Verification items for the finished model (mm, model axes). A direction names the side the tool comes from. Round coordinates to 2 decimals unless told otherwise and drop trailing zeros. Loops run counter-clockwise (first coordinate to the right, second up) from the corner with the lowest first, then second, coordinate; pieces in that order, holes last. Notation, with made-up numbers: M 84,-24 L 94,-24 A13 cw 94,-2 Z; hole C -12,64 d9. An arc over 180 degrees is marked long. One line per item, written item: value.
from build123d import *

# Parameters (mm, degrees)
SKETCH_1_W          = 23.4
SKETCH_1_H          = 12
SKETCH_1_R          = 1.75
SKETCH_1_R_2        = 1.6
SKETCH_1_R_3        = 1.15
EXTRUDE_1_DEPTH     = 1
EXTRUDE_START       = 1
SKETCH_1_4_W        = 23.4
SKETCH_1_4_H        = 12
EXTRUDE_2_DEPTH     = 3.1
SKETCH_3_R          = 0.35
CUT_EXTRUDE_3_DEPTH = 2
SKETCH_3_3_R        = 1
CUT_EXTRUDE_4_DEPTH = 1
SKETCH_3_4_R        = 0.8
CUT_EXTRUDE_5_DEPTH = 27.615221209


with BuildPart() as part:
    # 草图1 → 凸台-拉伸1 (new body)
    with BuildSketch(Plane(origin=(0, 0, 0), x_dir=(1, 0, 0), z_dir=(0, 1, 0))):
        with Locations((11.7, -6)):
            Rectangle(SKETCH_1_W, SKETCH_1_H)
        with Locations(Location((9.270831301, -3.4, 0), (0, 0, 270))):
            Circle(SKETCH_1_R, mode=Mode.SUBTRACT)
        with Locations(Location((9.270831301, -8.6, 0), (0, 0, 270))):
            Circle(SKETCH_1_R, mode=Mode.SUBTRACT)
        with Locations(Location((12.695740059, -6, 0), (0, 0, 270))):
            Circle(SKETCH_1_R_2, mode=Mode.SUBTRACT)
        with Locations(Location((18.395740059, -6, 0), (0, 0, 270))):
            Circle(SKETCH_1_R_3, mode=Mode.SUBTRACT)
    extrude(amount=EXTRUDE_1_DEPTH)

    # 草图1<4> → 凸台-拉伸2 (add)
    with BuildSketch(Plane(origin=(0, 0, 0), x_dir=(1, 0, 0), z_dir=(0, 1, 0)).offset(EXTRUDE_START)):
        with Locations((11.7, -6)):
            Rectangle(SKETCH_1_4_W, SKETCH_1_4_H)
        with BuildLine():
            ThreePointArc((9.300586178, -5.149747024), (7.876973085, -2.341860465), (10.964181547, -2.958338428))
            ThreePointArc((10.964181547, -2.958338428), (13.1957667, -2.53590223), (15.21679269, -3.572183362))
            ThreePointArc((15.21679269, -3.572183362), (19.67718661, -2.210818725), (22.395740059, -6))
            ThreePointArc((22.395740059, -6), (19.67718661, -9.789181275), (15.21679269, -8.427816638))
            ThreePointArc((15.21679269, -8.427816638), (13.1957667, -9.46409777), (10.964181547, -9.041661572))
            ThreePointArc((10.964181547, -9.041661572), (7.876973085, -9.658139535), (9.300586178, -6.850252976))
            ThreePointArc((9.300586178, -6.850252976), (9.195740059, -6), (9.300586178, -5.149747024))
        make_face(mode=Mode.SUBTRACT)
    extrude(amount=EXTRUDE_2_DEPTH)

    # 草图3 → 切除-拉伸3 (cut)
    with BuildSketch(Plane(origin=(0, 4.1, 0), x_dir=(1, 0, 0), z_dir=(0, 1, 0))):
        with Locations(Location((2.419185522, -2.108925173, 0), (0, 0, 270))):
            Circle(SKETCH_3_R)
        with Locations(Location((14.983521503, -1.209932246, 0), (0, 0, 270))):
            Circle(SKETCH_3_R)
        with Locations(Location((14.983521503, -10.376111281, 0), (0, 0, 270))):
            Circle(SKETCH_3_R)
        with Locations(Location((5.314681037, -6.384388153, 0), (0, 0, 270))):
            Circle(SKETCH_3_R)
    extrude(amount=-CUT_EXTRUDE_3_DEPTH, mode=Mode.SUBTRACT)

    # 草图3<3> → 切除-拉伸4 (cut)
    with BuildSketch(Plane(origin=(0, 4.1, 0), x_dir=(1, 0, 0), z_dir=(0, 1, 0))):
        with Locations(Location((1.568943185, -5.332489754, 0), (0, 0, 270))):
            Circle(SKETCH_3_3_R)
        with Locations(Location((2.419185522, -9.817518082, 0), (0, 0, 270))):
            Circle(SKETCH_3_3_R)
        with Locations((21.143175994, -2.108925173)):
            Circle(SKETCH_3_3_R)
        with Locations((21.143175994, -9.817518082)):
            Circle(SKETCH_3_3_R)
    extrude(amount=-CUT_EXTRUDE_4_DEPTH, mode=Mode.SUBTRACT)

    # 草图3<4> → 切除-拉伸5 (cut, through all)
    with BuildSketch(Plane(origin=(0, 4.1, 0), x_dir=(1, 0, 0), z_dir=(0, 1, 0))):
        with Locations(Location((1.568943185, -5.332489754, 0), (0, 0, 270))):
            Circle(SKETCH_3_4_R)
        with Locations(Location((21.143175994, -2.108925173, 0), (0, 0, 270))):
            Circle(SKETCH_3_4_R)
        with Locations(Location((2.419185522, -9.817518082, 0), (0, 0, 270))):
            Circle(SKETCH_3_4_R)
        with Locations(Location((21.143175994, -9.817518082, 0), (0, 0, 270))):
            Circle(SKETCH_3_4_R)
    extrude(amount=-CUT_EXTRUDE_5_DEPTH, mode=Mode.SUBTRACT)


solid = part.part
(1) Sectioned sample at A-A on z = 8. Enter the section's corners in (x, y).
Completed:
outline: M 0,0 L 7.63,0 L 7.63,4.1 L 0,4.1 Z; M 10.91,0 L 23.4,0 L 23.4,4.1 L 21.86,4.1 L 21.86,1 L 10.91,1 Z
(2) Mould release check, pull along X, two halves, no side actions. Record for faces 1 (the face through (2.96, 1.57, 9.23)), 2 (the face through (12, 2, 12)): +X half, -X half, draft (parallel to the pull), parting line (faces both ways), or undercut.
Completed:
face 1: undercut
face 2: draft
(3) Depth check by flat-ended pin: pin 1 Ø4 at (x, z) = (17.5, 7) entering from +Y. Enter the tip coordinate at first touch or a pass-through.
Completed:
pin 1: stops at y = 1
(4) Sectioned sample at B-B on x = 18. Enter the section's corners in (y, z), and give its area (3 significant figures).
Completed:
outline: M 0,0 L 4.1,0 L 4.1,2.02 L 1,2.02 L 1,4.92 L 0,4.92 Z; M 0,7.08 L 1,7.08 L 1,9.98 L 4.1,9.98 L 4.1,12 L 0,12 Z
area: 22.4 mm^2
(5) Thickness scan on L1, parallel to X at y = 0.45, z = 6; L2, parallel to Z at x = 8, y = 0.35; L3, parallel to Z at x = 7.75, y = 0.8. Record the ranges inside material, lowest first. Write a range as from..to.
Completed:
L1: x = 0..1.13, 2.01..11.1, 14.3..17.25, 19.55..23.4
L2: z = 0..2.2, 4.6..7.4, 9.8..12
L3: z = 0..2.53, 4.27..7.73, 9.47..12
(6) Tool access check on faces 3 (the face through (11.276, 0.493, 6.738)), 4 (the face through (13.23, 2.53, 9.46)). Record the directions out of +Z, -Z, +X, -X, +Y, -Y that give a thin tool (end or side, any length) a straight path to the whole face; none if there is none.
Completed:
face 3: +Y, -Y
face 4: +Y
(7) Sectioned sample at D-D on y = 3.8. Enter the section's corners in (x, z), and give its area (3 significant figures).
Completed:
outline: M 0,0 L 23.4,0 L 23.4,12 L 0,12 Z; hole C 1.57,5.33 d2; hole C 2.42,9.82 d2; hole C 2.42,2.11 d0.7; hole C 5.31,6.38 d0.7; hole M 9.3,5.15 A1.75 ccw long 10.96,2.96 A3.5 ccw 15.22,3.57 A4 ccw 20.2,2.43 A1 ccw long 21.16,3.11 A4 ccw 21.23,8.82 A1 ccw long 20.17,9.58 A4 ccw 15.22,8.43 A3.5 ccw 10.96,9.04 A1.75 ccw long 9.3,6.85 A3.5 ccw Z; hole C 14.98,1.21 d0.7; hole C 14.98,10.38 d0.7
area: 169 mm^2
(8) Sectioned sample at C-C on y = 1.5. Enter the section's corners in (x, z).
Completed:
outline: M 0,0 L 23.4,0 L 23.4,12 L 0,12 Z; hole C 1.57,5.33 d1.6; hole C 2.42,9.82 d1.6; hole M 9.3,5.15 A1.75 ccw long 10.96,2.96 A3.5 ccw 15.22,3.57 A4 ccw 20.52,2.61 A0.8 ccw long 20.88,2.86 A4 ccw 21.01,9.03 A0.8 ccw long 20.44,9.44 A4 ccw 15.22,8.43 A3.5 ccw 10.96,9.04 A1.75 ccw long 9.3,6.85 A3.5 ccw Z
